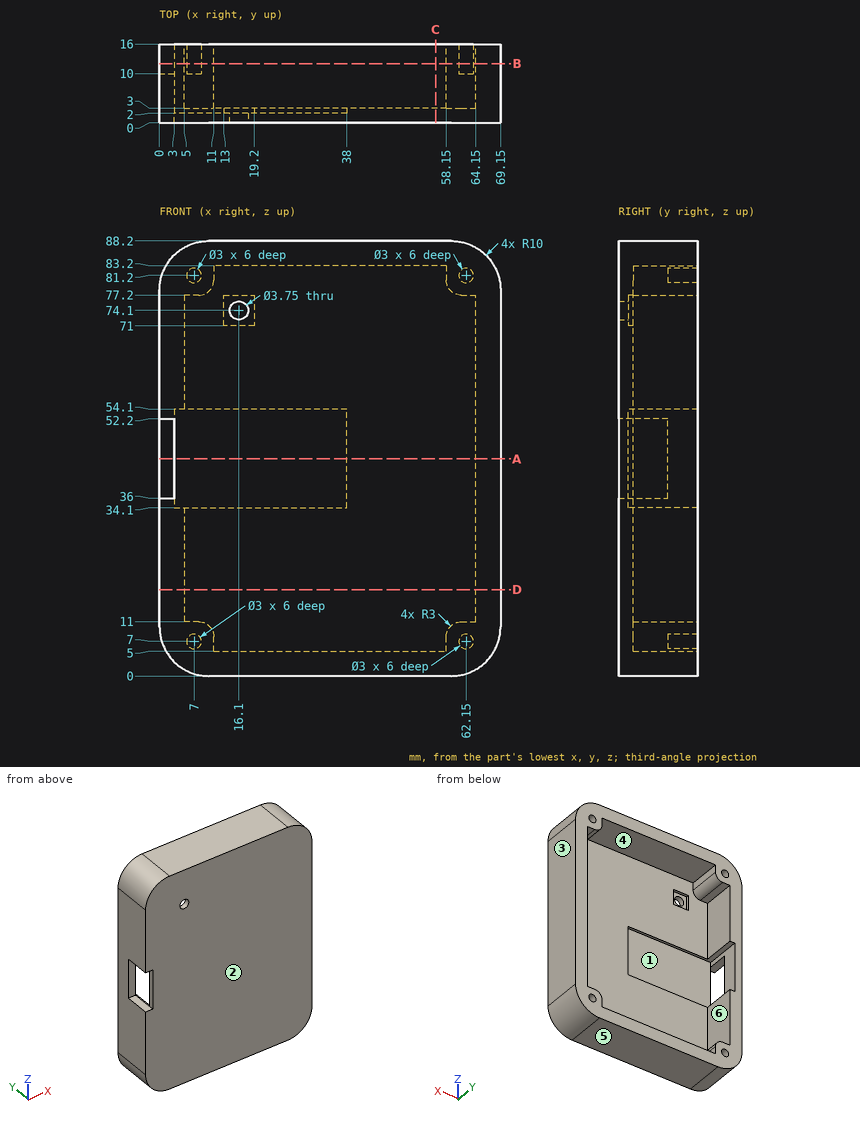
Study the drawing (mm; zero at the part's minimum x, y, z) and answer. A direction names the side the tool comes from. Round coordinates to 2 decimals unless told otherwise and drop trailing zeros. Order: outer loops, then holes, each group sorted by start corner. A loop starts at its lowest first (then second) coordinate and runs counter-clockwise, first axis right, second up. Notation, with made-up numbers: (76.25, 25.25) -> (104.25, 25.25) arc R17 cw to (104.25, 54.25) -> close; hole circle Ø8 at (81.5, 42.5). An arc over 180 degrees is marked (long way). Write each question's results on one line, items separated by ' | '. Start each with the question number.
Q1. Find section C-C (x = 56). Determine the outline of the cut face in (y, z).
Q2. Which of the six approach directions +Z, -Z, +X, -X, +Y, -Y give full straight-line access (tool end or side, diameter ignored) to the marked faces 1 and 2?
Q3. Each of these flat-tipped pins is pushed along its axis until it touches: pin 1 (3.5 mm diameter, centred on x = 7, y = 10, fed in from -Z); pin 2 (2.5 mm diameter, centred on x = 7, z = 7, fed in from +Y); pin 3 (8 mm diameter, centred on x = 16.5, z = 62, fed in from +Y). Where does it stop, or does it pass through?
Q4. Straight lines are drawn through the part: probe 1 along X at (y, z) = (9.5, 72); probe 2 along Z at (x, y) = (35, 4.5); probe 3 along X at (y, z) = (11.8, 7). For each, find the intervals that lie inside material, in ascending order. Write a range as from..to.
Q5. The mould has two halves that part along X. Classify the marked faces 3, 4, 5 and 6: pulls with the +X half, pulls with the -X half, needs draft (parallel to the pull), parting line crosses it, or undercut.
Q6. Find section A-A (z = 44). Determine the outline of the cut face in (x, y), then the cut area to 3 significant figures.
Q7. Find section B-B (y = 12). Give the number of separate pieces and of enclosed holes in the cut face, then the cut area to 3 significant figures.
Q8. Find section D-D (z = 17.5). Determine the outline of the cut face in (x, y), then the cut area to 3 significant figures.
Worked answers:
1) outline: (0, 0) -> (16, 0) -> (16, 5) -> (3, 5) -> (3, 83.2) -> (16, 83.2) -> (16, 88.2) -> (0, 88.2) -> close
2) face 1: +Y | face 2: +Z, -Z, +X, -X, -Y
3) pin 1: stops at z = 0.08 | pin 2: stops at y = 10 | pin 3: stops at y = 3
4) probe 1: x = 0..5, 64.15..69.15 | probe 2: z = 0..5, 83.2..88.2 | probe 3: x = 0.46..5.5, 8.5..11, 58.15..60.65, 63.65..68.69
5) face 3: pulls with the +X half | face 4: undercut | face 5: needs draft | face 6: undercut
6) outline: (0, 10) -> (3, 10) -> (3, 16) -> (0, 16) -> close; (3, 0) -> (69.15, 0) -> (69.15, 16) -> (64.15, 16) -> (64.15, 3) -> (38, 3) -> (38, 2) -> (3, 2) -> close | area: 246 mm2
7) separate pieces: 1 | enclosed holes: 5 | area: 1,460 mm2
8) outline: (0, 0) -> (69.15, 0) -> (69.15, 16) -> (64.15, 16) -> (64.15, 3) -> (5, 3) -> (5, 16) -> (0, 16) -> close | area: 337 mm2
